Design review of the part built by this model. Coordinates are the model's own, in mm. Round coordinates to 2 decimals unless told otherwise and drop trailing zeros. Write each loop counter-clockwise with the first axis right and the second up, starting at its lowest first coordinate (ties: lowest second). Pieces come first, ordered by that corner, then holes. Notation, with made-up numbers: (65.25, 12) -> (76.25, 12) arc R5 ccw to (76.25, 18) -> close; hole circle Ø8 at (48, 38.5). An arc over 180 degrees is marked (long way). Write item = value, one per line. Start each with the question number.
Item 1: For pin 1 Ø4.5 at (x, y) = (42.33, -26.28) entering from +Z, flat-tipped, find the tip position at first contact; note if it passes through.
Item 2: Add section A-A, the plane y = 6.35. State the section outline as (x, z) points.
Item 3: To check wall thickness, follow L1, parallel to X at y = -26.5, z = 3.75; L2, parallel to X at y = -1, z = 4; L3, parallel to X at y = 8, z = 2.75. State the ranges of each line that lie inside material, in increasing order.
from build123d import *

# Parameters (mm, degrees)
F0_W     = 127
F0_H     = 152.4
F0_R     = 3.175
F0_R_2   = 2.38125
F0_W_2   = 25.4
F1_DEPTH = 6.35


with BuildPart() as f1:
    # F0 (on Top) → F1 (new body)
    with BuildSketch(Plane.XY):
        with Locations((-14.822774, -0.883641)):
            Rectangle(F0_W, F0_H)
        with Locations((-67.210274, -65.971141)):
            Circle(F0_R, mode=Mode.SUBTRACT)
        with Locations((-20.602145, -67.558641)):
            Circle(F0_R_2, mode=Mode.SUBTRACT)
        with Locations((-4.727145, -67.558641)):
            Circle(F0_R_2, mode=Mode.SUBTRACT)
        with Locations((40.739726, -67.558641)):
            Circle(F0_R_2, mode=Mode.SUBTRACT)
        with Locations((42.327226, -26.283641)):
            Circle(F0_R_2, mode=Mode.SUBTRACT)
        with Locations((-71.972774, 6.35)):
            Circle(F0_R_2, mode=Mode.SUBTRACT)
        with Locations((-59.272774, 6.35)):
            Circle(F0_R_2, mode=Mode.SUBTRACT)
        with Locations((-67.210274, 64.203859)):
            Circle(F0_R, mode=Mode.SUBTRACT)
        with Locations((42.327226, 49.916359)):
            Circle(F0_R_2, mode=Mode.SUBTRACT)
        with Locations((61.377226, -0.883641)):
            Rectangle(F0_W_2, F0_H)
        with Locations((56.614726, -67.558641)):
            Circle(F0_R_2, mode=Mode.SUBTRACT)
        with Locations((55.027226, -26.283641)):
            Circle(F0_R_2, mode=Mode.SUBTRACT)
        with Locations((62.964726, -0.883641)):
            Circle(F0_R, mode=Mode.SUBTRACT)
        with Locations((55.027226, 49.916359)):
            Circle(F0_R_2, mode=Mode.SUBTRACT)
    extrude(amount=F1_DEPTH)


solid = f1.part
Result set:
q1.pin_1 = through
q2.outline = (-78.32, 0) -> (-74.35, 0) -> (-74.35, 6.35) -> (-78.32, 6.35) -> close; (-69.59, 0) -> (-61.65, 0) -> (-61.65, 6.35) -> (-69.59, 6.35) -> close; (-56.89, 0) -> (74.08, 0) -> (74.08, 6.35) -> (-56.89, 6.35) -> close
q3.L1 = -78.32 to 39.96, 44.7 to 52.66, 57.4 to 74.08
q3.L2 = -78.32 to 59.79, 66.14 to 74.08
q3.L3 = -78.32 to -73.69, -70.26 to -60.99, -57.56 to 74.08
